Build history of the part. All positions in model axes, mm. Face numbers are marked on the shaded views. A direction names the side the tool comes from. Coordinates: 2 decimals unless noted, no trailing zeros. Order: outer loops, then holes, each group sorted by start corner. A loop starts at its lowest first (then second) coordinate and runs counter-clockwise, first axis right, second up. Notation, with made-up numbers: (38, 22.25) - (88, 22.25) arc R27 cw to (88, 53.25) - close; hole circle Ø7 at (85.25, -13.75). An arc over 180 degrees is marked (long way). Return JSON: item names as keys, results as strings.
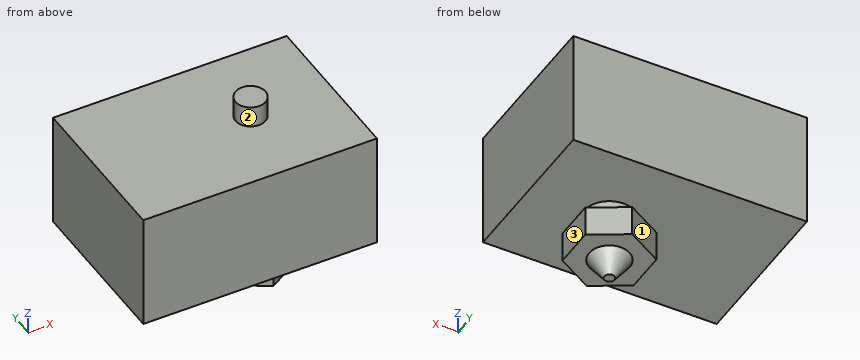
from build123d import *

# Parameters (mm, degrees)
F0_R     = 1.475
F1_DEPTH = 2.1
F0_W     = 23
F0_H     = 16
F2_DEPTH = 11.5
F3_R     = 2.5
F4_DEPTH = 1.5
F6_DEPTH = 3
F7_R     = 2
F9_R     = 0.5


with BuildPart() as f1:
    # F0 (on Top) → F1 (new body)
    with BuildSketch(Plane.XY):
        Circle(F0_R)
    extrude(amount=F1_DEPTH)

    # F0 (on Top) → F2 (join)
    with BuildSketch(Plane.XY):
        with Locations((-3.5, 0)):
            Rectangle(F0_W, F0_H)
        Circle(F0_R, mode=Mode.SUBTRACT)
        Circle(F0_R)
    extrude(amount=-F2_DEPTH)

    # F3 (on face) → F4 (join)
    with BuildSketch(Plane(origin=(0, 0, -11.5), x_dir=(1, 0, 0), z_dir=(0, 0, -1))):
        Circle(F3_R)
    extrude(amount=F4_DEPTH)

    # F5 (on face) → F6 (join)
    with BuildSketch(Plane(origin=(0, 0, -13), x_dir=(1, 0, 0), z_dir=(0, 0, -1))):
        Polygon((3.5, -2.0207259422), (3.5, 2.0207259422), (0, 4.0414518843), (-3.5, 2.0207259422), (-3.5, -2.0207259422), (0, -4.0414518843), align=None)
    extrude(amount=F6_DEPTH)

    # F7 (on face) → F10 section 0
    with BuildSketch(Plane(origin=(0, 0, -16), x_dir=(1, 0, 0), z_dir=(0, 0, -1))):
        Circle(F7_R)
    # F9 (on offset) → F10 section 1
    with BuildSketch(Plane(origin=(0, 0, -18), x_dir=(1, 0, 0), z_dir=(0, 0, -1))):
        Circle(F9_R)
    loft()


solid = f1.part
1. Probe L1, parallel to Z at x = -10.75, y = -3.5; L2, parallel to X at y = 2, z = -14; L3, parallel to Y at x = 1, z = -17. List the from-to ranges inside material, lowest first.
Check values:
{"L1": "-11.5 to 0", "L2": "-3.5 to 3.5", "L3": "-0.75 to 0.75"}
2. Tool access for the marked faces 1, 2 and 3: list every direction of +Z, -Z, +X, -X, +Y, -Y with a clear straight run to the whole face (end or side of a thin tool).
Check values:
{"face 1": "-Z, -X, +Y", "face 2": "+Z", "face 3": "-Z, +X, +Y, -Y"}
3. Drop flat-ended pins along their axis: pin 1 (5 mm diameter, centred on x = 2, y = 3.5, fed in from -Z); pin 2 (2 mm diameter, centred on x = -0.5, y = 1.5, fed in from -Z); pin 3 (0.9 mm diameter, centred on y = -0.5, z = -14.5, fed in from -X). Give the stop position or say it passes through.
Check values:
{"pin 1": "z = -16.63", "pin 2": "z = -17.89", "pin 3": "x = -3.5"}
4. Cut at B-B on z = -13.75. Give the cut face in (x, y).
Check values:
{"outline": "(-3.5, -2.02) - (0, -4.04) - (3.5, -2.02) - (3.5, 2.02) - (0, 4.04) - (-3.5, 2.02) - close"}
5. Cut at C-C on x = -10.5. Give the cut face in (y, z), plus the area to 3 significant figures.
Check values:
{"outline": "(-8, -11.5) - (8, -11.5) - (8, 0) - (-8, 0) - close", "area": "184 mm²"}
6. Cut at A-A on y = -3. Give the cut face in (x, z).
Check values:
{"outline": "(-15, -11.5) - (8, -11.5) - (8, 0) - (-15, 0) - close; (-1.8, -16) - (1.8, -16) - (1.8, -13) - (-1.8, -13) - close"}
